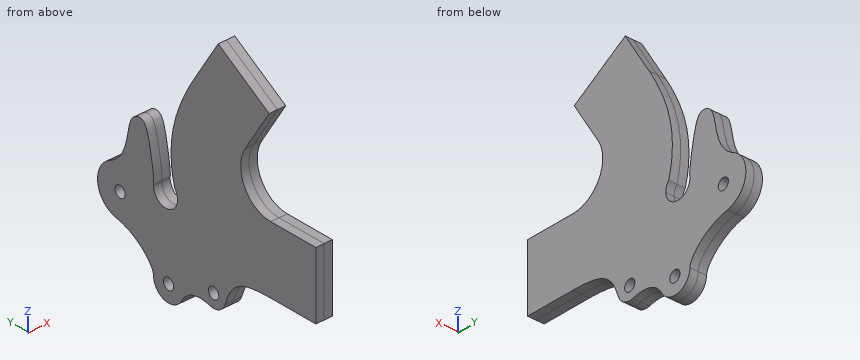
Autodesk Inventor part; units mm, degrees
ref_plane "YZ Plane" through (0, 0, 0) normal (1, 0, 0) x (0, 1, 0)
ref_plane "XZ Plane" through (0, 0, 0) normal (0, 1, 0) x (-1, 0, 0)
ref_plane "XY Plane" through (0, 0, 0) normal (0, 0, 1) x (1, 0, 0)
ref_plane "Plano de trabajo1" through (-185.7873, -389.4877, 168.7004) normal (1, 0, 0) x (0, 1, 0)
sketch "Boceto1" plane through (-185.7873, -389.4877, 168.7004) normal (1, 0, 0) x (0, 1, 0)
  spline S0 degree 3 poles (534.733, 23.2998) (534.7105, 23.7942) (534.6906, 24.2218) (534.6565, 24.9274) (534.6425, 25.2033) (534.6129, 25.7399) (534.6044, 25.8219) (534.6094, 25.4554) (534.6229, 25.0104) (534.6701, 23.6469) (534.7034, 22.7415) (534.7857, 20.5852) (534.8338, 19.3549) (534.9389, 16.7287) (534.9948, 15.3579) (535.1069, 12.6551) (535.1621, 11.3489) (535.2644, 8.9741) (535.3106, 7.9282) (535.3879, 6.2371) (535.4183, 5.608) (535.4589, 4.8538) (535.4688, 4.7358) (535.4667, 5.0314) (535.4548, 5.4422) (535.4103, 6.7433) (535.3782, 7.6213) (535.2979, 9.7332) (535.2505, 10.9469) (535.1465, 13.5533) (535.0909, 14.9211) (534.9787, 17.6317) (534.9233, 18.9486) (534.8197, 21.3576) (534.7727, 22.4265) (534.733, 23.2998) knots -6.594944 -6.594944 -6.594944 -6.594944 -6.363484 -6.363484 -6.132024 -6.132024 -5.723223 -5.723223 -5.314421 -5.314421 -4.90562 -4.90562 -4.496818 -4.496818 -4.088016 -4.088016 -3.679215 -3.679215 -3.270413 -3.270413 -2.861611 -2.861611 -2.45281 -2.45281 -2.044008 -2.044008 -1.635207 -1.635207 -1.226405 -1.226405 -0.817603 -0.817603 -0.408802 -0.408802 0 0 0 0 construction
  spline S1 degree 3 poles (563.9582, 57.2503) (564.369, 57.506) (564.6982, 57.7109) (565.1814, 58.0114) (565.334, 58.1062) (565.502, 58.21) (565.3211, 58.0968) (564.4035, 57.5239) (563.6756, 57.0698) (561.7633, 55.8774) (560.5973, 55.1504) (557.9767, 53.5169) (556.5472, 52.6259) (553.6106, 50.7959) (552.1317, 49.8744) (549.319, 48.122) (548.0121, 47.3078) (545.7443, 45.8954) (544.8051, 45.3106) (543.4219, 44.4496) (542.9911, 44.1816) (542.6995, 44.001) (542.8416, 44.0901) (543.6854, 44.617) (544.379, 45.0497) (546.2318, 46.2051) (547.3731, 46.9167) (549.9574, 48.5276) (551.3756, 49.4116) (554.3045, 51.2368) (555.7872, 52.1607) (558.622, 53.9269) (559.9471, 54.7524) (562.2635, 56.1952) (563.2327, 56.7987) (563.9582, 57.2503) knots -8.403752 -8.403752 -8.403752 -8.403752 -8.108809 -8.108809 -7.813866 -7.813866 -7.292942 -7.292942 -6.772017 -6.772017 -6.251093 -6.251093 -5.730168 -5.730168 -5.209244 -5.209244 -4.68832 -4.68832 -4.167395 -4.167395 -3.646471 -3.646471 -3.125546 -3.125546 -2.604622 -2.604622 -2.083698 -2.083698 -1.562773 -1.562773 -1.041849 -1.041849 -0.520924 -0.520924 0 0 0 0 construction
  spline S2 degree 3 poles (534.6356, 25.8056) (534.6632, 25.2036) (534.6939, 24.5175) (534.7607, 23.0024) (534.7966, 22.178) (534.9005, 19.7543) (534.9715, 18.0684) (535.1144, 14.6095) (535.185, 12.8696) (535.3167, 9.5648) (535.3764, 8.0315) (535.4771, 5.3755) (535.517, 4.2783) (535.5717, 2.669) (535.5858, 2.1723) (535.5862, 1.8506) (535.5724, 2.0287) (535.5185, 3.0427) (535.4789, 3.869) (535.3787, 6.0669) (535.3192, 7.4176) (535.1878, 10.4704) (535.1173, 12.1433) (534.9744, 15.5937) (534.9034, 17.3383) (534.7703, 20.6697) (534.7095, 22.2248) (534.6062, 24.9384) (534.5647, 26.071) (534.5067, 27.7605) (534.4907, 28.3011) (534.4865, 28.7134) (534.4984, 28.5811) (534.5489, 27.6545) (534.5869, 26.869) (534.6356, 25.8056) knots -8.403752 -8.403752 -8.403752 -8.403752 -8.108809 -8.108809 -7.813866 -7.813866 -7.292942 -7.292942 -6.772017 -6.772017 -6.251093 -6.251093 -5.730168 -5.730168 -5.209244 -5.209244 -4.68832 -4.68832 -4.167395 -4.167395 -3.646471 -3.646471 -3.125546 -3.125546 -2.604622 -2.604622 -2.083698 -2.083698 -1.562773 -1.562773 -1.041849 -1.041849 -0.520924 -0.520924 0 0 0 0 construction
  line L0 (525, 5.254) -> (525, 25.254)
  line L1 (525, 25.254) -> (540, 25.254)
  arc A0 (540, 25.254) -> (548.4852, 40.5618) centre (540, 35.2596) ccw
  line L2 (548.4852, 40.5618) -> (540.5364, 53.2825)
  line L3 (540.5364, 53.2825) -> (557.4974, 63.8809)
  line L4 (557.4974, 63.8809) -> (565.4462, 51.1602)
  line L5 (525, 15.254) -> (575, 17.0001) construction
  line L6 (549.0169, 58.5817) -> (575, 17.0001) construction
  line L7 (525, 5.254) -> (540, 5.254)
  circle A1 centre (575, 17.0001) radius 4 construction
  line L8 (565.4462, 51.1602) -> (573.2852, 38.6152) construction
  line L9 (573.8755, 23.7788) -> (571.0024, 16.8605) construction
  spline S3 degree 4 poles (565.4462, 51.1602) (573.2852, 38.6152) (573.8755, 31.3158) (573.8755, 23.7788) (571.0024, 16.8605) knots 1 1 1 1 1 2 2 2 2 2
  circle A2 centre (575, 17.0001) radius 4
  line L10 (578.9765, 17.4327) -> (578.7688, 19.3424) construction
  line L11 (578.7688, 19.3424) -> (580.8115, 30.4088) construction
  line L12 (580.8115, 30.4088) -> (581.5561, 33.9943) construction
  line L13 (581.5561, 33.9943) -> (588.3082, 32.4831) construction
  line L14 (588.3082, 32.4831) -> (587.0334, 24.49) construction
  line L15 (587.0334, 24.49) -> (590.1956, 18.7656) construction
  line L16 (546.3222, 5.254) -> (540, 5.254) construction
  line L17 (573.2852, 38.6152) -> (573.8755, 31.3158) construction
  line L18 (573.8755, 31.3158) -> (573.8755, 23.7788) construction
  arc A3 (591.5375, 3.1103) -> (593.375, 17.2458) centre (590.1405, 10.4791) ccw
  arc A4 (569.6718, -8.8556) -> (579.02, -6.402) centre (574.02, -6.3872) ccw
  arc A5 (555.1918, -3.2238) -> (560.0425, -5.8618) centre (559, -2) ccw
  spline S4 degree 4 poles (578.9765, 17.4327) (578.7688, 19.3424) (580.8115, 30.4088) (581.5561, 33.9943) (588.3082, 32.4831) (587.0334, 24.49) (590.1956, 18.7656) (593.375, 17.2458) knots 0 0 0 0 0 1 2 3 4 4 4 4 4
  line L19 (590.1956, 18.7656) -> (593.375, 17.2458) construction
  spline S5 degree 4 poles (555.1918, -3.2238) (553.3097, 2.6327) (551.1077, 4.616) (546.3222, 5.254) (540, 5.254) knots 21.570729 21.570729 21.570729 21.570729 21.570729 22 22 22 22 22
  line L20 (555.1918, -3.2238) -> (553.3097, 2.6327) construction
  line L21 (553.3097, 2.6327) -> (551.1077, 4.616) construction
  line L22 (551.1077, 4.616) -> (546.3222, 5.254) construction
  line L23 (569.6718, -8.8556) -> (566.9184, -4.0055) construction
  line L24 (566.9184, -4.0055) -> (560.0425, -5.8618) construction
  spline S6 degree 2 poles (569.6718, -8.8556) (566.9184, -4.0055) (560.0425, -5.8618) knots 1 1 1 2 2 2
  line L25 (575, 17.0001) -> (528.8996, 17.0001) construction
  line L26 (591.5375, 3.1103) -> (584.136, 1.7072) construction
  line L27 (584.136, 1.7072) -> (579.0273, -3.9321) construction
  line L28 (579.0273, -3.9321) -> (579.02, -6.402) construction
  spline S7 degree 3 poles (591.5375, 3.1103) (584.136, 1.7072) (579.0273, -3.9321) (579.02, -6.402) knots 1 1 1 1 2 2 2 2
  point P0 (389.4877, -168.7004)
  point P1 (534.733, 23.2998)
  point P2 (563.9582, 57.2503)
  point P3 (534.6356, 25.8056)
  point P4 (571.974, 19.6161)
  point P5 (578.9765, 17.4332)
  point P6 (571.0024, 16.8605)
  dimension "d78" = 8
  dimension "d75" = 20
  dimension "d76" = 60
  dimension "d77" = 15
  dimension "d232" = 15
  dimension "d233" = 10
  dimension "d234" = 8
  dimension "d290" = 2
  dimension "d291" = 50
extrude "Extrusión1" add sketch "Boceto1" along normal mid plane 5 contours L0 L1 A0 L2 L3 L4 S3 A2 S4 A3 S7 A4 S6 A5 S5 L7
sketch "Boceto2" plane through (-188.2873, -389.4877, 168.7004) normal (-1, 0, 0) x (0, 0, 1)
  arc A0 (-5.8618, 560.0425) -> (-3.2238, 555.1918) centre (-2, 559) ccw
  arc A1 (-6.402, 579.02) -> (-8.8556, 569.6718) centre (-6.3872, 574.02) ccw
  arc A2 (17.2458, 593.375) -> (3.1103, 591.5375) centre (10.4791, 590.1405) ccw
  point P0 (-168.7004, 389.4877)
hole "Agujero1" at (-188.2873, 169.5123, 166.7004) at (-188.2873, 184.5323, 162.3132) at (-188.2873, 200.6529, 179.1795) direction (1, 0, 0) diameter 3.4 end through all
properties part number "soporte_eje_trasero"
Geometry: final body of the model. Coordinates: model frame, mm. Coordinates: 2 decimals unless noted, no trailing zeros. Order: outer loops, then holes, each group sorted by start corner. A loop starts at its lowest first (then second) coordinate and runs counter-clockwise, first axis right, second up. Notation, with made-up numbers: M 38,83 L 88,83 A23 ccw 88,122 Z; hole C 41,-1.75 d6. An arc over 180 degrees is marked long. One line per question, with ' | ' between items. Start each with the question number.
Item 1: Cut plane C-C, the plane x = -187.1. Count the separate pieces of the cut face and the enclosed holes in it, then the cut area to 3 significant figures.
Item 2: Cut plane B-B, the plane y = 149. Return the cut outline in (x, z).
Item 3: Pin query (flat end, axial travel): pin 1 Ø1.2 at (x, y) = (-187, 141.5) entering from -Z; pin 2 Ø0.8 at (x, y) = (-187, 141.5) entering from +Z; pin 3 Ø2 at (y, z) = (169.51, 166.7) entering from -X; pin 4 Ø2 at (x, z) = (-184.5, 168) entering from -Y. Return the tip coordinate at first contact, or that it passes through.
Item 4: Cut plane D-D, the plane z = 227. Return the cut outline in (x, y).
Item 5: Cut plane A-A, the plane z = 183.5. Return the cut outline in (x, y), then the cut area to 3 significant figures.
Item 6: Ray query, probe 1 along Y at (x, z) = (-187.7, 201); probe 2 along Z at (x, y) = (-183.7, 185.5); probe 3 along Z at (x, y) = (-183.8, 143.5). Return the intervals inside material, ascending. Write a range as [from, to].
A:
1) separate pieces: 1 | enclosed holes: 3 | area: 2,500 mm2
2) outline: M -188.29,173.95 L -183.29,173.95 L -183.29,193.95 L -188.29,193.95 Z
3) pin 1: stops at z = 173.95 | pin 2: stops at z = 193.95 | pin 3: passes through | pin 4: stops at y = 164.24
4) outline: M -188.29,159.08 L -183.29,159.08 L -183.29,171.5 L -188.29,171.5 Z
5) outline: M -188.29,135.51 L -183.29,135.51 L -183.29,182.17 L -188.29,182.17 Z; M -188.29,188.85 L -183.29,188.85 L -183.29,206.78 L -188.29,206.78 Z | area: 323 mm2
6) probe 1: y = [160.07, 183.45], [192.75, 195.85] | probe 2: z = [157.41, 160.92], [163.71, 181.7] | probe 3: z = [173.95, 193.95]
